Design review of the part built by this model. Coordinates are the model's own, in mm. Face numbers are marked on the shaded views. Coordinates: 2 decimals unless noted, no trailing zeros. Loops run counter-clockwise (first coordinate to the right, second up) from the corner with the lowest first, then second, coordinate; pieces in that order, holes last. Notation, with made-up numbers: M 3.5,-16.75 L 61.5,-16.75 A15 ccw 61.5,-6.75 Z; hole C 12,-22 d8. An arc over 180 degrees is marked long. One line per item, written item: value.
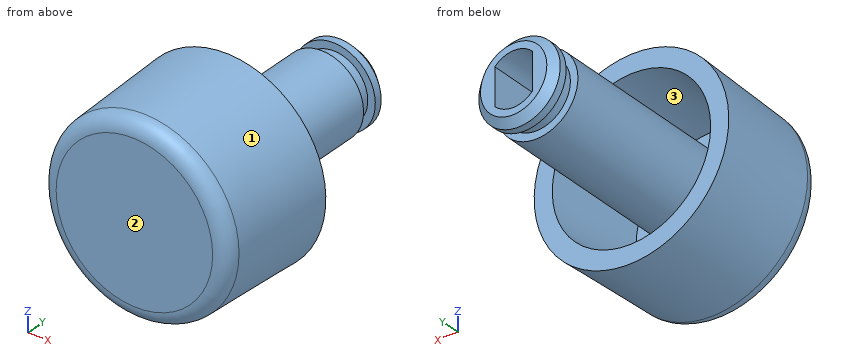
Autodesk Inventor part; units mm, degrees
ref_plane "YZ Plane" through (0, 0, 0) normal (1, 0, 0) x (0, 1, 0)
ref_plane "XZ Plane" through (0, 0, 0) normal (0, 1, 0) x (-1, 0, 0)
ref_plane "XY Plane" through (0, 0, 0) normal (0, 0, 1) x (1, 0, 0)
sketch "Эскиз1" plane through (0, 0, 0) normal (1, 0, 0) x (0, 1, 0)
  line L0 (0, 0) -> (35, 0)
  line L1 (0, 0) -> (0, 6.15)
  line L2 (0, 6.15) -> (7.9944, 6.45)
  line L3 (7.9944, 6.45) -> (7.9944, 5.25)
  line L4 (7.9944, 5.25) -> (1.2, 4.995)
  line L5 (1.2, 4.995) -> (1.2, 2.7)
  line L6 (18, 2.7) -> (18, 0)
  line L7 (16, 2.7) -> (16, 2.2)
  line L8 (16, 2.2) -> (17, 2.2)
  line L9 (17, 2.2) -> (17, 2.7)
  line L10 (18, 2.7) -> (17, 2.7)
  line L11 (16, 2.7) -> (1.2, 2.7)
  point P0 (0, 3.075)
  dimension "d0" = 35
  dimension "d1" = 6.15
  dimension "d2" = 8
  dimension "d4" = 18
  dimension "d5" = 2.7
  dimension "d6" = 6.45
  dimension "d7" = 1.2
  dimension "d8" = 1.2
  dimension "d11" = 1
  dimension "d12" = 1
  dimension "d21" = 0.5
  dimension "d22" = 0
revolve "Вращение1" add sketch "Эскиз1" angle 360 about axis through (0, 0, 0) along (0, 1, 0)
fillet "Сопряжение1" radius 1 1 edges at (0, 0, -6.15)
sketch "Эскиз2" plane through (0, 18, 0) normal (0, 1, 0) x (1, 0, 0)
  circle A0 centre (0, 0) radius 1.75
  line L0 (-1.25, 1.2247) -> (-1.25, -1.2247)
  line L1 (1.25, 1.2247) -> (1.25, -1.2247)
  dimension "d13" = 3.5
  dimension "d19" = 1.25
  dimension "d20" = 1.25
extrude "Выдавливание1" cut sketch "Эскиз2" against normal blind 16 contours L1 A0 L0
chamfer "Фаска1" distance 0.5 angle 45 1 edges at (0, 18, -2.7)
properties part number "Кнопка для кухонной плиты (Укороченная)"
(1) Mouldability with a two-part tool opening along X and no side actions: class the marked faces 1, 2 and 3 as released by +X, released by -X, zero draft, split by the parting line, or undercut.
Reply:
face 1: split by the parting line
face 2: zero draft
face 3: undercut
(2) To check wall thickness, follow line 1 along X through (y, z) = (4.5, -0.25); line 2 along Z through (x, y) = (-0.25, 7.5); line 3 along X through (y, z) = (14.5, -0.5). State the ranges of each line that lie inside material, in increasing order. Write a range as [from, to].
Reply:
line 1: x = [-6.31, -5.11], [-2.69, -1.25], [1.25, 2.69], [5.11, 6.31]
line 2: z = [-6.43, -5.23], [-2.69, -1.73], [1.73, 2.69], [5.23, 6.43]
line 3: x = [-2.65, -1.25], [1.25, 2.65]
(3) We need section B-B on y = 11. State the section outline as (x, z) points.
Reply:
outline: C 0,0 d5.4; hole M -1.25,-1.22 A1.75 ccw 1.25,-1.22 L 1.25,1.22 A1.75 ccw -1.25,1.22 Z
(4) Insertion check: pin 1 (3 mm diameter, centred on x = 0.5, z = 0.5, fed in from +Y); pin 2 (2 mm diameter, centred on y = 12, z = -0.5, fed in from -X); pin 3 (2.5 mm diameter, centred on y = 10.5, z = 0, fed in from +X); pin 4 (5 mm diameter, centred on x = 4.5, y = 2.5, fed in from -Z). Each pin has a flat end and moves straight along its axis. Give the tip position at first contact, or say it passes through.
Reply:
pin 1: stops at y = 18
pin 2: stops at x = -2.7
pin 3: stops at x = 2.7
pin 4: stops at z = -5.92
